```python
from build123d import *

# Parameters (mm, degrees)
F0_R     = 7.85
F2_DEPTH = 6
F3_D     = 8.78
F4_SIZE  = 1


with BuildPart() as f2:
    # F0 (on Front) → F2 (new body)
    with BuildSketch(Plane.XZ):
        Circle(F0_R)
    extrude(amount=F2_DEPTH)

    # F3 (through all)
    with Locations(Plane(origin=(0, 0, 0), x_dir=(1, 0, 0), z_dir=(0, 1, 0))):
        with Locations((0, 0)):
            Hole(F3_D / 2)

    # F4
    f4_edges = [f2.edges().sort_by_distance(p)[0] for p in [
        (-7.85, -6, 0),
    ]]
    chamfer(f4_edges, length=F4_SIZE)


solid = f2.part
```
Input: part model. Units: mm. Frame: model coordinates. Coordinates: 2 decimals unless noted, no trailing zeros. Loops run counter-clockwise (first coordinate to the right, second up) from the corner with the lowest first, then second, coordinate; pieces in that order, holes last. Notation, with made-up numbers: M 83.25,68 L 141.25,68 A14 cw 141.25,82 Z; hole C 81,-39.75 d5. An arc over 180 degrees is marked long. One line per item, written item: value.
(1) Section C-C (y = -5.45). Output: boundary loops of the cut face in (x, z).
Filled in:
outline: C 0,0 d14.8; hole C 0,0 d8.78
(2) Section D-D (y = -4.05). Output: boundary loops of the cut face in (x, z), and give its area (3 significant figures).
Filled in:
outline: C 0,0 d15.7; hole C 0,0 d8.78
area: 133 mm^2
(3) Pull-direction query (Z, two-part tool) for faces 1 (the flat face through (3.4, 0, -3.4)), 2 (the cylindrical face through (-5.786, -2.465, 5.305)), 3 (the cylindrical face through (0.571, -3.042, -4.353)); classes: +Z half, -Z half, draft (parallel to the pull), parting line (faces both ways), or undercut.
Filled in:
face 1: draft
face 2: parting line
face 3: undercut
(4) Section B-B (z = 0). Output: boundary loops of the cut face in (x, y).
Filled in:
outline: M -7.85,-5 L -6.85,-6 L -4.39,-6 L -4.39,0 L -7.85,0 Z; M 4.39,-6 L 6.85,-6 L 7.85,-5 L 7.85,0 L 4.39,0 Z
(5) Line query: line 1 along Z through (x, y) = (0, -2.25); line 2 along X through (y, z) = (-1.35, -3). Output: solid intervals per line, ascending. Write a range as from..to.
Filled in:
line 1: -7.85..-4.39, 4.39..7.85
line 2: -7.25..-3.21, 3.21..7.25
(6) Pin query (flat end, axial travel): pin 1 (1.5 mm diameter, centred on x = 3.5, y = -3, fed in from +Z); pin 2 (1.5 mm diameter, centred on y = -1.5, z = -3, fed in from +X); pin 3 (2 mm diameter, centred on y = -4.5, z = 4.5, fed in from +X). Return the tip coordinate at first contact, or that it passes through.
Filled in:
pin 1: z = 7.35
pin 2: x = 7.52
pin 3: x = 7.03
(7) Section A-A (x = 0). Output: boundary loops of the cut face in (y, z).
Filled in:
outline: M -6,-6.85 L -5,-7.85 L 0,-7.85 L 0,-4.39 L -6,-4.39 Z; M -6,4.39 L 0,4.39 L 0,7.85 L -5,7.85 L -6,6.85 Z
